Could you check a few things on this model? Use its own coordinates, in mm. A direction names the side the tool comes from. Round coordinates to 2 decimals unless told otherwise and drop trailing zeros. Loops run counter-clockwise (first coordinate to the right, second up) from the corner with the lowest first, then second, coordinate; pieces in that order, holes last. Notation, with made-up numbers: (0.5, 50) - (28.5, 50) arc R24 ccw to (28.5, 87) - close; hole circle Ø7 at (76, -24.5). An arc over 180 degrees is marked (long way). Use one line per item in the form item = value.
```python
from build123d import *

# Parameters (mm, degrees)
BOSS_EXTRUDE1_DEPTH = 25
SKETCH2_W           = 42
SKETCH2_H           = 22
CUT_EXTRUDE1_DEPTH  = 30.5
SKETCH3_W           = 42
SKETCH3_H           = 22
CUT_EXTRUDE2_DEPTH  = 30.5
FILLET1_R           = 10
FILLET2_R           = 5
FILLET3_R           = 5
SKETCH5_W           = 10
SKETCH5_H           = 5
CUT_EXTRUDE3_DEPTH  = 30.5
SKETCH6_W           = 10
SKETCH6_H           = 10
CUT_EXTRUDE4_DEPTH  = 30.5


with BuildPart() as part:
    # Sketch1 → Boss-Extrude1 (new body)
    with BuildSketch(Plane(origin=(0, 0, 0), x_dir=(1, 0, 0), z_dir=(0, 1, 0))):
        Polygon((-23.5, -15.5), (-35.5, -15.5), (-35.5, -18.5), (0, -18.5), (35.5, -18.5), (35.5, -15.5), (23.5, -15.5), (23.5, 18.5), (50, 18.5), (50, 87.5), (16, 87.5), (16, 99.5), (13, 99.5), (13, 28.5), (-23.5, 28.5), align=None)
    extrude(amount=BOSS_EXTRUDE1_DEPTH)

    # Sketch2 → Cut-Extrude1 (cut)
    with BuildSketch(Plane.XY.offset(18.5)):
        with Locations((0, 12.5)):
            Rectangle(SKETCH2_W, SKETCH2_H)
    extrude(amount=-CUT_EXTRUDE1_DEPTH, mode=Mode.SUBTRACT)

    # Sketch3 → Cut-Extrude2 (cut)
    with BuildSketch(Plane.ZY.offset(-13)):
        with Locations((-64.067301197, 12.5)):
            Rectangle(SKETCH3_W, SKETCH3_H)
    extrude(amount=-CUT_EXTRUDE2_DEPTH, mode=Mode.SUBTRACT)

    # Fillet1
    fillet1_edges = [part.edges().sort_by_distance(p)[0] for p in [
        (16, 12.5, -87.5),
        (50, 12.5, -18.5),
        (23.5, 12.5, -18.5),
        (-23.5, 12.5, 15.5),
        (23.5, 12.5, 15.5),
    ]]
    fillet(fillet1_edges, radius=FILLET1_R)

    # Fillet2
    fillet2_edges = [part.edges().sort_by_distance(p)[0] for p in [
        (-23.5, 12.5, -28.5),
    ]]
    fillet(fillet2_edges, radius=FILLET2_R)

    # Fillet3
    fillet3_edges = [part.edges().sort_by_distance(p)[0] for p in [
        (50, 12.5, -87.5),
    ]]
    fillet(fillet3_edges, radius=FILLET3_R)

    # Sketch5 → Cut-Extrude3 (cut)
    with BuildSketch(Plane.ZY.offset(-21)):
        with Locations((-5.5, 9.426274429)):
            Rectangle(SKETCH5_W, SKETCH5_H)
        with Locations((-5.5, 14.426274429)):
            Rectangle(SKETCH5_W, SKETCH5_H)
    extrude(amount=-CUT_EXTRUDE3_DEPTH, mode=Mode.SUBTRACT)

    # Sketch6 → Cut-Extrude4 (cut)
    with BuildSketch(Plane(origin=(0, 0, -43.067301197), x_dir=(-1, 0, 0), z_dir=(0, 0, -1))):
        with Locations((-37, 12.54801)):
            Rectangle(SKETCH6_W, SKETCH6_H)
    extrude(amount=-CUT_EXTRUDE4_DEPTH, mode=Mode.SUBTRACT)


solid = part.part
```
1. If we section it at B-B, the plane x = 27.5: Write out the boundary of the cut face in (y, z), plus the area to 3 significant figures.
Solution:
outline = (0, -87.5) - (25, -87.5) - (25, -16.5) - (0, -16.5) - close; (0, 13.5) - (25, 13.5) - (25, 18.5) - (0, 18.5) - close; hole (1.5, -85.07) - (23.5, -85.07) - (23.5, -43.07) - (1.5, -43.07) - close
area = 976 mm^2
2. On a 3-axis mill with a long thin cutter (end or side, diameter ignored), from which of +Z, -Z, +X, -X, +Y, -Y can I reach the whole of each face in a straight line? I mean faces 1 (the face through (22, 6.926, -6)), 2 (the face through (0, 1, 18.5)), 3 (the face through (48.5, 12.68, -86.07)), 4 (the face through (37, 21, -18.5)), 5 (the face through (28, 12, -85.067)). Say none if no direction works.
Solution:
face_1 = +X
face_2 = +Z, +X, -X, +Y, -Y
face_3 = -Z, +X, +Y, -Y
face_4 = +X, +Y, -Y
face_5 = -X
3. If we section it at A-A, the plane y = 15: Count the separate pieces of the cut face and the enclosed holes in it, plus the area to 3 significant figures.
Solution:
separate_pieces = 3
enclosed_holes = 0
area = 1,990 mm^2
4. We'd pull the mould along X, two halves only. Please class faces 6 (the face through (43.5, 13, -64)), 7 (the face through (36, 12, -87.5)), 8 (the face through (-21, 12, 3)): +X half, -X half, draft (parallel to the pull), parting line (faces both ways), or undercut.
Solution:
face_6 = -X half
face_7 = draft
face_8 = undercut
5. If we section it at D-D, the plane x = 18.5: Write out the boundary of the cut face in (y, z).
Solution:
outline = (0, -90.89) - (25, -90.89) - (25, 18.5) - (23.5, 18.5) - (23.5, -12) - (1.5, -12) - (1.5, 18.5) - (0, 18.5) - close; hole (1.5, -85.07) - (23.5, -85.07) - (23.5, -43.07) - (1.5, -43.07) - close
6. Please list where these lines run through material, in increasing order: line 1 along Z through (x, y) = (34, 5.75); line 2 along Z through (x, y) = (34.5, 12.5); line 3 along Y through (x, z) = (33.5, -75).
Solution:
line_1 = -87.5 to -85.07, -43.07 to -18.5, 15.5 to 18.5
line_2 = -87.5 to -85.07, 15.5 to 18.5
line_3 = 0 to 1.5, 23.5 to 25
7. For P1, Ø10, axis at y = 12, z = -18.5, coming from the +X side; P2, Ø4, axis at x = 22, y = 7, coming from the -Z side; P3, Ø6, axis at x = -21.5, y = 17.5, coming from the -Z side, each with a flat end and sliding along its axis, tell me the tip position at first contact or that it passes through.
Solution:
P1 = 48.66
P2 = -89.5
P3 = -28.5
